from build123d import *
from build123d import SkipClean  # not in build123d's __all__

# Parameters (mm, degrees)
F0_R     = 19.05
F1_DEPTH = 12.7
F2_R     = 12.573
F3_DEPTH = 50.8


with BuildPart() as f1:
    # F0 (on Right) → F1 (new body)
    with BuildSketch(Plane.YZ):
        Circle(F0_R)
    extrude(amount=F1_DEPTH)

    # F2 (on face) → F3 (join)
    with BuildSketch(Plane.YZ.offset(12.7)):
        Circle(F2_R)
    extrude(amount=F3_DEPTH)

    # F4 (on Front) → F5 (revolve, cut)
    with BuildSketch(Plane.XZ):
        with BuildLine():
            Line((69.85, -12.7), (69.85, 12.7))
            ThreePointArc((69.85, 12.7), (57.15, 0), (69.85, -12.7))
        make_face()
    with SkipClean():  # cleaning this boolean's faces spoils the solid; the shape is the same uncleaned
        revolve(axis=Axis((69.85, 0, 17.1570373535), (0, 0, 1)), mode=Mode.SUBTRACT)


solid = f1.part
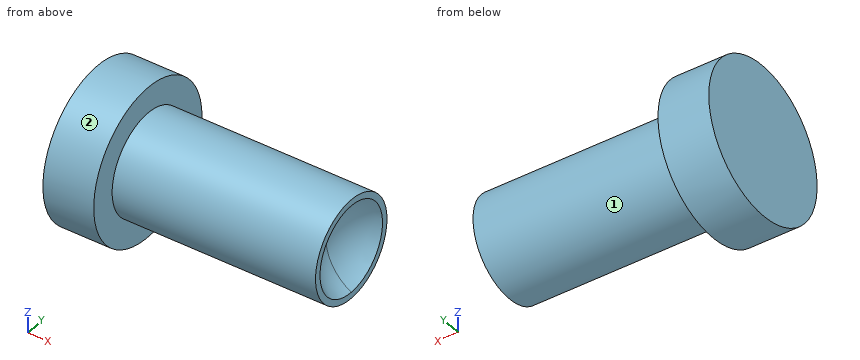
Geometry: final body of the model. Coordinates: model frame, mm. Face numbers are marked on the shaded views. A direction names the side the tool comes from. Give positions to 0.01 mm unless a question says otherwise; leave off trailing zeros. Write each loop counter-clockwise with the first axis right and the second up, starting at its lowest first coordinate (ties: lowest second). Pieces come first, ordered by that corner, then holes. Notation, with made-up numbers: M -2.5,7 L 10.5,7 A20 cw 10.5,19 Z; hole C 67.5,26 d6. An arc over 180 degrees is marked long. Answer in a Markdown table with one row per item. Add a question column.
(1) Reachability of the marked faces 1 and 2 from +Z, -Z, +X, -X, +Y, -Y: full face, straight path, thin tool, end or side. Return the list, or none.
(2) Section B-B on y = 16. Return loops of the section in (x, z), and give its area (3 significant figures).
(3) Section D-D on x = 9.5. Return loops of the section in (y, z).
(4) Section C-C on z = 15.5. Return loops of the section in (x, y).
(5) Section A-A on x = 44. Return loops of the section in (y, z), and give its area (3 significant figures).
(6) First-contact query: pin 1 (2 mm diameter, centred on x = 16, z = 3.5, fed in from +Y); pin 2 (1.5 mm diameter, centred on x = 25, z = -11, fed in from +Y); pin 3 (12 mm diameter, centred on x = 10.5, y = -5.5, fed in from -Z); pin 4 (3 mm diameter, centred on x = 29, y = 14.5, fed in from -Z). Flat tips, straight axial feed; report the tip coordinate or a pass-through.
(7) Ray query, line 1 (X direction, y = 11, z = -8); line 2 (Z direction, x = 18, y = 0.5); line 3 (Z direction, x = 4, y = -0.5). Return the intervals inside material, ascending.
Result set:
| question | item | result |
|---|---|---|
| 1 | face 1 | +X |
| 1 | face 2 | +X, -X |
| 2 | outline | M 0,-10.34 L 12.7,-10.34 L 12.7,10.34 L 0,10.34 Z |
| 2 | area | 263 mm^2 |
| 3 | outline | C 0,0 d38.1 |
| 4 | outline | M 0,-11.07 L 12.7,-11.07 L 12.7,11.07 L 0,11.07 Z |
| 5 | outline | C 0,0 d25.15 |
| 5 | area | 497 mm^2 |
| 6 | pin 1 | stops at y = 12.32 |
| 6 | pin 2 | stops at y = 7.28 |
| 6 | pin 3 | stops at z = -19.05 |
| 6 | pin 4 | passes through |
| 7 | line 1 | x = 0 to 12.7 |
| 7 | line 2 | z = -12.56 to 12.56 |
| 7 | line 3 | z = -19.04 to 19.04 |
